Could you check a few things on this model? Use its own coordinates, in mm. Face numbers are marked on the shaded views. A direction names the side the tool comes from. Give positions to 0.01 mm unless a question says otherwise; leave off trailing zeros. Order: outer loops, then holes, each group sorted by start corner. A loop starts at its lowest first (then second) coordinate and runs counter-clockwise, first axis right, second up. Notation, with made-up numbers: (-24.75, 43) -> (-0.75, 43) arc R27 cw to (-0.75, 68) -> close; hole circle Ø10 at (51.5, -3). An arc over 180 degrees is marked (long way). One line per item, written item: value.
```python
from build123d import *

# Parameters (mm, degrees)
SKETCH1_R           = 75
BOSS_EXTRUDE1_DEPTH = 10
SKETCH2_R           = 22.5
BOSS_EXTRUDE2_DEPTH = 50
CUT_EXTRUDE1_DEPTH  = 30
CUT_EXTRUDE2_DEPTH  = 118.260394038
SKETCH5_R           = 12.5
CUT_EXTRUDE3_DEPTH  = 122.86057607


with BuildPart() as part:
    # Sketch1 → Boss-Extrude1 (new body)
    with BuildSketch(Plane.XY):
        Circle(SKETCH1_R)
    extrude(amount=BOSS_EXTRUDE1_DEPTH)

    # Sketch2 → Boss-Extrude2 (add)
    with BuildSketch(Plane.XY.offset(10)):
        Circle(SKETCH2_R)
    extrude(amount=BOSS_EXTRUDE2_DEPTH)

    # Sketch3 → Cut-Extrude1 (cut, symmetric)
    with BuildSketch(Plane(origin=(0, 0, 0), x_dir=(1, 0, 0), z_dir=(0, 1, 0))):
        with BuildLine():
            Line((6, -40), (6, -60))
            ThreePointArc((6, -60), (0, -66), (-6, -60))
            Line((-6, -60), (-6, -40))
            ThreePointArc((-6, -40), (0, -34), (6, -40))
        make_face()
    extrude(amount=CUT_EXTRUDE1_DEPTH, both=True, mode=Mode.SUBTRACT)

    # Sketch4 → Cut-Extrude2 (cut, through all)
    with BuildSketch(Plane.XY.offset(10)):
        with BuildLine():
            ThreePointArc((37.476659403, 37.476659403), (0, 53), (-37.476659403, 37.476659403))
            ThreePointArc((-37.476659403, 37.476659403), (-47.376154339, 37.476659403), (-47.376154339, 47.376154339))
            ThreePointArc((-47.376154339, 47.376154339), (0, 67), (47.376154339, 47.376154339))
            ThreePointArc((47.376154339, 47.376154339), (47.376154339, 37.476659403), (37.476659403, 37.476659403))
        make_face()
    extrude(amount=-CUT_EXTRUDE2_DEPTH, mode=Mode.SUBTRACT)

    # Sketch5 → Cut-Extrude3 (cut, through all)
    with BuildSketch(Plane.XY.offset(60)):
        Circle(SKETCH5_R)
    extrude(amount=-CUT_EXTRUDE3_DEPTH, mode=Mode.SUBTRACT)


solid = part.part
```
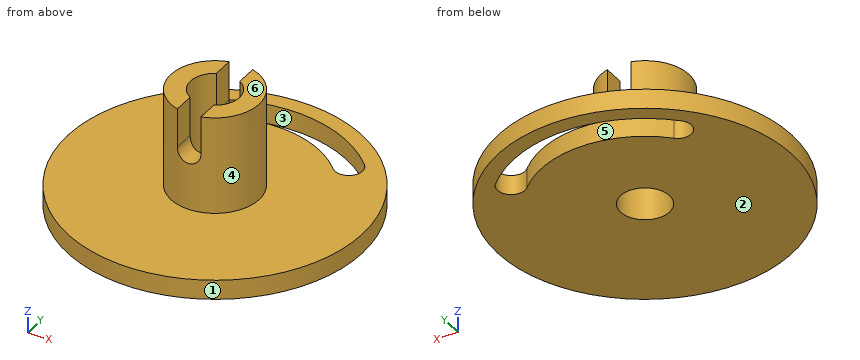
1) For the marked faces 4, 5 and 6, which set-ups out of +Z, -Z, +X, -X, +Y, -Y let a thin tool reach every point of the face, with its end or its side?
Answer below:
face 4: +Z
face 5: +Z, -Z
face 6: +Z, +X, -X, +Y, -Y
2) If I drill on line 1 along Y through (x, z) = (0, 18); line 2 along Z through (x, y) = (-40, -25); line 3 along Y through (x, z) = (-30, 9.5), over which ranges is the centre line in solid material (lowest first)?
Answer below:
line 1: y = -22.5 to -12.5, 12.5 to 22.5
line 2: z = 0 to 10
line 3: y = -68.74 to 43.69, 59.91 to 68.74
3) Suppose I cut it at D-D, the plane z = 24. Write out the boundary of the cut face in (x, y).
Answer below:
outline: circle Ø45 at (0, 0); hole circle Ø25 at (0, 0)
4) For P1, Ø2, axis at y = -4, z = 31.5, coming from the +X side; P2, Ø5, axis at x = -13.5, z = 24, coming from the -Y side; P3, Ø3, axis at y = -17.5, z = 49.5, coming from the -X side, each with a flat end and sliding along its axis, tell me the tip position at first contact or that it passes through.
Answer below:
P1: stops at x = 22.3
P2: stops at y = -19.63
P3: stops at x = -15.82
5) Suppose I cut it at C-C, the plane y = 0. Write out the boundary of the cut face in (x, z).
Answer below:
outline: (-75, 0) -> (-12.5, 0) -> (-12.5, 60) -> (-22.5, 60) -> (-22.5, 10) -> (-75, 10) -> close; (12.5, 0) -> (75, 0) -> (75, 10) -> (22.5, 10) -> (22.5, 60) -> (12.5, 60) -> close
6) Suppose I cut it at B-B, the plane z = 47. Write out the boundary of the cut face in (x, y).
Answer below:
outline: (-6, -21.69) -> (-6, -10.97) arc R12.5 cw to (-6, 10.97) -> (-6, 21.69) arc R22.5 ccw to start; (6, -21.69) arc R22.5 ccw to (6, 21.69) -> (6, 10.97) arc R12.5 cw to (6, -10.97) -> close
7) Suppose I cut it at A-A, the plane x = 0. Write out the boundary of the cut face in (y, z), then the cut area to 3 significant figures.
Answer below:
outline: (-75, 0) -> (-12.5, 0) -> (-12.5, 34) -> (-22.5, 34) -> (-22.5, 10) -> (-75, 10) -> close; (12.5, 0) -> (53, 0) -> (53, 10) -> (22.5, 10) -> (22.5, 34) -> (12.5, 34) -> close; (67, 0) -> (75, 0) -> (75, 10) -> (67, 10) -> close
area: 1,590 mm2
8) We'd pull the mould along Y, two halves only. Please class the marked faces 1, 2 and 3: +Y half, -Y half, draft (parallel to the pull), parting line (faces both ways), or undercut.
Answer below:
face 1: parting line
face 2: draft
face 3: undercut
